```python
from build123d import *

# Parameters (mm, degrees)
F0_R     = 9.5
F1_DEPTH = 240
F3_W     = 80
F3_H     = 45.5118790269
F4_DEPTH = 5
F6_D     = 3.3


with BuildPart() as f1:
    # F0 (on Front) → F1 (new body)
    with BuildSketch(Plane.XZ):
        Circle(F0_R)
    extrude(amount=F1_DEPTH)

    # F3 (on offset) → F4 (cut)
    with BuildSketch(Plane.YZ.offset(9.5)):
        with Locations((-40, 0.18652156)):
            Rectangle(F3_W, F3_H)
    extrude(amount=-F4_DEPTH, mode=Mode.SUBTRACT)

    # F6 (through all)
    with Locations(Plane.YZ.offset(4.5)):
        with Locations((-47, 0), (-5, 0)):
            Hole(F6_D / 2)


solid = f1.part
```
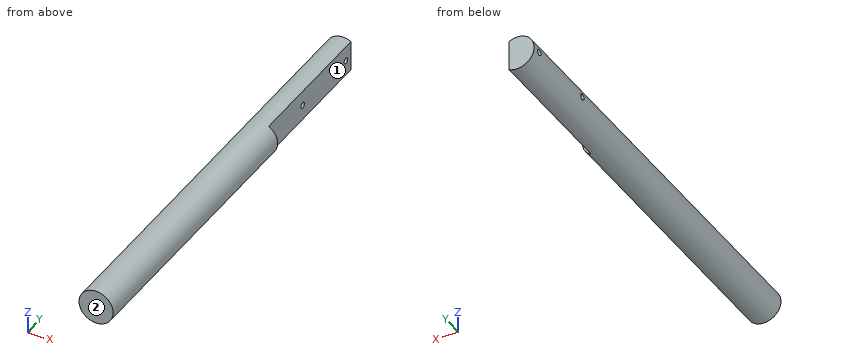
Verification items for the finished model (mm, model axes). Face numbers are marked on the shaded views. A direction names the side the tool comes from. Give positions to 0.01 mm unless a question says otherwise; leave off trailing zeros. Loops run counter-clockwise (first coordinate to the right, second up) from the corner with the lowest first, then second, coordinate; pieces in that order, holes last.
1. Section check C-C, the plane z = -6.25. Enter the section's corners in (x, y).
2. Section check B-B, the plane y = -140.5. Enter the section's corners in (x, z).
3. Thickness scan on line 1 (Y direction, x = 1, z = 0); line 2 (Z direction, x = -4.5, y = -47); line 3 (Z direction, x = 0.25, y = -47). Record the ranges inside material, lowest first.
4. Section check A-A, the plane x = -5.5. Enter the section's corners in (y, z).
5. Set-up check for the marked faces 1 and 2: record each of +Z, -Z, +X, -X, +Y, -Y from which the full face is reachable in a straight line by a thin tool's end or side.
6. Go/stop test with flat-tipped pins: pin 1 Ø5 at (x, y) = (-5.5, -119.5) entering from +Z; pin 2 Ø4 at (x, z) = (6, -1) entering from +Y; pin 3 Ø3 at (y, z) = (-25.5, -1.5) entering from +X; pin 4 Ø5 at (x, y) = (-6.5, -127.5) entering from -Z. Record where each tip stops, or that it passes through.
7. Section check D-D, the plane y = -67. Enter the section's corners in (x, z).
Geometry says:
1. outline: (-7.15, -240) - (7.15, -240) - (7.15, -80) - (4.5, -80) - (4.5, 0) - (-7.15, 0) - close
2. outline: circle Ø19 at (0, 0)
3. line 1: y = -240 to -48.65, -45.35 to -6.65, -3.35 to 0
3. line 2: z = -8.37 to -1.65, 1.65 to 8.37
3. line 3: z = -9.5 to -1.65, 1.65 to 9.5
4. outline: (-240, -7.75) - (0, -7.75) - (0, 7.75) - (-240, 7.75) - close; hole circle Ø3.3 at (-47, 0); hole circle Ø3.3 at (-5, 0)
5. face 1: +Z, -Z, +X, +Y
5. face 2: +Z, -Z, +X, -X, -Y
6. pin 1: stops at z = 9.01
6. pin 2: stops at y = 0
6. pin 3: stops at x = 4.5
6. pin 4: stops at z = -8.62
7. outline: (4.5, -8.37) - (4.5, 8.37) arc R9.5 ccw (long way) to start
